CAD build for the part. Positions are in the model's coordinates, mm. A direction names the side the tool comes from. Round coordinates to 2 decimals unless told otherwise and drop trailing zeros. Loops run counter-clockwise (first coordinate to the right, second up) from the corner with the lowest first, then second, coordinate; pieces in that order, holes last.
```python
from build123d import *

# Parameters (mm, degrees)
F0_W     = 70.2332556248
F0_H     = 17.4792334437
F0_W_2   = 11.8431299925
F1_DEPTH = 25
F0_H_2   = 68.3041326702
F2_DEPTH = 25
F3_W     = 12.7824991941
F3_H     = 73.9819798619
F4_DEPTH = 25


with BuildPart() as f1:
    # F0 (on Front) → F1 (new body)
    with BuildSketch(Plane.XZ):
        with Locations((-3.1356401742, 42.5850078464)):
            Rectangle(F0_W, F0_H)
        with Locations((37.9025526345, 42.5850078464)):
            Rectangle(F0_W_2, F0_H)
    extrude(amount=F1_DEPTH)

    # F0 (on Front) → F2 (join)
    with BuildSketch(Plane.XZ):
        with Locations((37.9025526345, -0.3066752106)):
            Rectangle(F0_W_2, F0_H_2)
        with Locations((37.9025526345, 42.5850078464)):
            Rectangle(F0_W_2, F0_H)
    extrude(amount=F2_DEPTH)

    # F3 (on Front) → F4 (join)
    with BuildSketch(Plane.XZ):
        with Locations((-27.5457836688, 14.2613416538)):
            Rectangle(F3_W, F3_H)
    extrude(amount=F4_DEPTH)


solid = f1.part
```
Item 1: Cut at D-D, the plane x = -29. Give the cut face in (y, z), plus the area to 3 significant figures.
Answers follow:
outline: (-25, -22.73) - (0, -22.73) - (0, 51.32) - (-25, 51.32) - close
area: 1,850 mm2
Item 2: Flat gauge pins, fed straight in: P1, Ø14, axis at x = -26.5, y = -17.5, coming from the -Z side; P2, Ø6, axis at y = -5, z = 22, coming from the -X side. Where does each tip first touch, or does it go through?
Answers follow:
P1: stops at z = -22.73
P2: stops at x = -33.94
Item 3: Cut at C-C, the plane x = 30. Give the cut face in (y, z), plus the area to 3 significant figures.
Answers follow:
outline: (-25, 33.85) - (0, 33.85) - (0, 51.32) - (-25, 51.32) - close
area: 437 mm2
Item 4: Cut at A-A, the plane z = 5. Give the cut face in (x, y), plus the area to 3 significant figures.
Answers follow:
outline: (-33.94, -25) - (-21.15, -25) - (-21.15, 0) - (-33.94, 0) - close; (31.98, -25) - (43.82, -25) - (43.82, 0) - (31.98, 0) - close
area: 616 mm2
Item 5: Probe line 1 (X direction, y = -17.25, z = 29); line 2 (Z direction, x = -15.5, y = -12.75); line 3 (Z direction, x = -21.5, y = -13). List the from-to ranges inside material, lowest first.
Answers follow:
line 1: x = -33.94 to -21.15, 31.98 to 43.82
line 2: z = 33.85 to 51.32
line 3: z = -22.73 to 51.32
Item 6: Cut at B-B, the plane y = -3. Give the cut face in (x, z), plus the area to 3 significant figures.
Answers follow:
outline: (-38.25, 33.85) - (-33.94, 33.85) - (-33.94, -22.73) - (-21.15, -22.73) - (-21.15, 33.85) - (31.98, 33.85) - (31.98, -34.46) - (43.82, -34.46) - (43.82, 51.32) - (-38.25, 51.32) - close
area: 2,970 mm2
Item 7: 3-axis set-ups, long thin cutter, end or side, ignore diameter. For faces 4 (the flat face through (-36, -12, 33.845)), 5 (the flat face through (43.824, -12, 8)), 6 (the flat face through (5, -12, 33.845)): which of +Z, -Z, +X, -X, +Y, -Y reach the whole face in a straight line?
Answers follow:
face 4: -Z, -X, +Y, -Y
face 5: +Z, -Z, +X, +Y, -Y
face 6: -Z, +Y, -Y
Item 8: Two-plate mould, pull along X, no slides. Class faces 1 (the flat face through (-33.937, -12, 5)), 2 (the flat face through (38, -12, -34.459)), 3 (the flat face through (-21.155, -12, 5)): released by +X, released by -X, zero draft, split by the parting line, or undercut.
Answers follow:
face 1: released by -X
face 2: zero draft
face 3: undercut
